Source: CAD feature listing. Evaluate the final solid. Frame: model axes, mm. Round coordinates to 2 decimals unless told otherwise and drop trailing zeros. Loops run counter-clockwise (first coordinate to the right, second up) from the corner with the lowest first, then second, coordinate; pieces in that order, holes last.
Item 1: Ray query, L1, parallel to Z at x = -2.55, y = -0.25; L2, parallel to X at y = 2, z = 29.5; L3, parallel to Y at x = -0.2, z = -168. Return the intervals inside material, ascending.
Item 2: Section query A-A on x = 0. Return loops of the section in (y, z) (1 decimal).
Item 3: First-contact query: P1, Ø1.5, axis at x = -2, y = -1.5, coming from the -Z side. Flat tip, straight axial feed; report the tip coordinate or a pass-through.
Item 4: Section query C-C on z = -96.5. Return loops of the section in (x, y), then the cut area to 3 significant figures.
Item 5: Section query D-D on z = 26.5. Return loops of the section in (x, y), then the cut area to 3 significant figures.
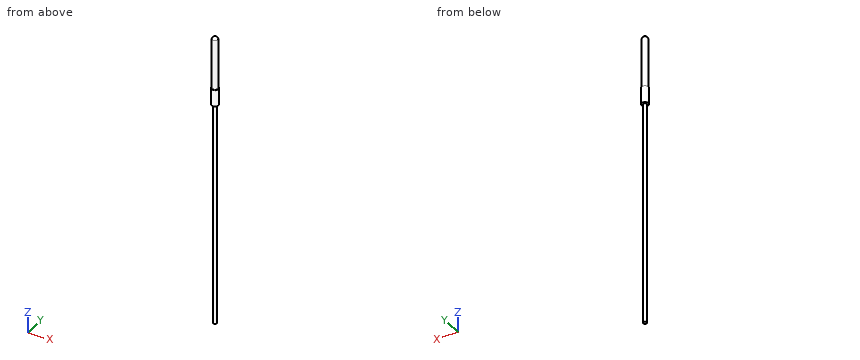
```python
from build123d import *

# Parameters (mm, degrees)
ESQUISSE1_R        = 2.5
BOSS_EXTRU_1_DEPTH = 45
D_ME1_FACE_RADIUS  = 2.5
D_ME1_HEIGHT       = 2
ESQUISSE2_R        = 3
BOSS_EXTRU_2_DEPTH = 15
ESQUISSE3_R        = 1.5
BOSS_EXTRU_3_DEPTH = 200


with BuildPart() as part:
    # Esquisse1 → Boss.-Extru.1 (new body)
    with BuildSketch(Plane.XY):
        with Locations(Location((0, 0, 0), (0, 0, 180))):
            Circle(ESQUISSE1_R)
    extrude(amount=BOSS_EXTRU_1_DEPTH)

    # Dôme1: a dome of height H over a round flat face of radius A is a cap of a sphere of radius (A * A + H * H) / (2 * H)
    d_me1_r = (D_ME1_FACE_RADIUS * D_ME1_FACE_RADIUS + D_ME1_HEIGHT * D_ME1_HEIGHT) / (2 * D_ME1_HEIGHT)
    d_me1_base = Plane((0, 0, 45), z_dir=(0, 0, 1))
    with Locations(d_me1_base.offset(D_ME1_HEIGHT - d_me1_r)):
        d_me1_ball = Sphere(d_me1_r, mode=Mode.PRIVATE)
    add(split(d_me1_ball, bisect_by=d_me1_base, keep=Keep.TOP, mode=Mode.PRIVATE))

    # Esquisse2 → Boss.-Extru.2 (add)
    with BuildSketch(Plane(origin=(0, 0, 0), x_dir=(-1, 0, 0), z_dir=(0, 0, -1))):
        with Locations(Location((0, 0, 0), (0, 0, 180))):
            Circle(ESQUISSE2_R)
    extrude(amount=BOSS_EXTRU_2_DEPTH)

    # Esquisse3 → Boss.-Extru.3 (add)
    with BuildSketch(Plane(origin=(0, 0, -15), x_dir=(-1, 0, 0), z_dir=(0, 0, -1))):
        Circle(ESQUISSE3_R)
    extrude(amount=BOSS_EXTRU_3_DEPTH)


solid = part.part
```
Data:
1. L1: z = -15 to 0
1. L2: x = -1.5 to 1.5
1. L3: y = -1.49 to 1.49
2. outline: (-3, -15) - (-1.5, -15) - (-1.5, -215) - (1.5, -215) - (1.5, -15) - (3, -15) - (3, 0) - (2.5, 0) - (2.5, 45) arc R2.6 ccw to (-2.5, 45) - (-2.5, 0) - (-3, 0) - close
3. P1: stops at z = -15
4. outline: circle Ø3 at (0, 0)
4. area: 7.07 mm2
5. outline: circle Ø5 at (0, 0)
5. area: 19.6 mm2
